from build123d import *

# Parameters (mm, degrees)
F1_DEPTH = 482.6
F2_R     = 22.9562722026
F3_DEPTH = 25.4


# Not quite as in the source:
# - a feature names something its author has since deleted; it is built from what else it names


with BuildPart() as f1:
    # F0 (on Right) → F1 (new body)
    with BuildSketch(Plane.YZ):
        with BuildLine():
            Line((-812.6182556152, 512.6869344869), (-812.6182556152, 611.3093582153))
            Line((-812.6182556152, 611.3093582153), (-825.3182556152, 611.3093582153))
            Line((-825.3182556152, 611.3093582153), (-825.3182556152, 510.914683342))
            ThreePointArc((-825.3182556152, 510.914683342), (-828.5785642638, 501.8659167533), (-836.8610188459, 496.9760562897))
            Line((-836.8610188459, 496.9760562897), (-938.4610188459, 496.9760562897))
            Line((-938.4610188459, 496.9760562897), (-938.4610188459, 484.2760562897))
            Line((-938.4610188459, 484.2760562897), (-840.6965225196, 484.2760562897))
            ThreePointArc((-840.6965225196, 484.2760562897), (-822.0453350188, 489.7370832304), (-812.6182556152, 506.7317819438))
            ThreePointArc((-812.6182556152, 506.7317819438), (-812.7921868823, 509.7093582153), (-812.6182556152, 512.6869344869))
        make_face()
    extrude(amount=F1_DEPTH)

    # F2 (on Right) → F3 (join)
    with BuildSketch(Plane.YZ):
        with Locations((-826.0604739189, 499.5044767857)):
            Circle(F2_R)
    extrude(amount=F3_DEPTH)


solid = f1.part
The model under review builds one solid part; all positions refer to its coordinate system, in mm. A direction names the side the tool comes from. Coordinates: 2 decimals unless noted, no trailing zeros. Order: outer loops, then holes, each group sorted by start corner. A loop starts at its lowest first (then second) coordinate and runs counter-clockwise, first axis right, second up. Notation, with made-up numbers: (-11, 1) -> (44, 1) arc R29 cw to (44, 30) -> close; hole circle Ø3 at (8.25, -36.5). An arc over 180 degrees is marked (long way). Answer in a Markdown table with one row per item.
(1) Machinability: for faces 1 (the flat face through (238, -938.461, 491)), 2 (the flat face through (25.4, -837, 510)), which of the approach directions +Z, -Z, +X, -X, +Y, -Y give a long, thin tool a straight path to every point of the face, cutting with its end or side? Answer none if there is none.
Answers:
| item | result |
|---|---|
| face 1 | +Z, -Z, +X, -X, -Y |
| face 2 | +Z, +X, -Y |
(2) Insertion check: pin 1 (3 mm diameter, centred on x = 188, z = 578, fed in from -Y); pin 2 (3 mm diameter, centred on x = 112, y = -870, fed in from -Z); pin 3 (8 mm diameter, centred on x = 218, z = 507, fed in from +Y). Each pin has a flat end and moves straight along its axis. Give the tip position at first contact, or say it passes through.
Answers:
| item | result |
|---|---|
| pin 1 | y = -825.32 |
| pin 2 | z = 484.28 |
| pin 3 | y = -812.62 |
(3) Consider section A-A (x = 370.5). Write out the cut boundary in (y, z).
Answers:
| item | result |
|---|---|
| outline | (-938.46, 484.28) -> (-840.7, 484.28) arc R25.57 ccw to (-812.62, 506.73) arc R25.57 cw to (-812.62, 512.69) -> (-812.62, 611.31) -> (-825.32, 611.31) -> (-825.32, 510.91) arc R14.19 cw to (-836.86, 496.98) -> (-938.46, 496.98) -> close |
(4) Consider section B-B (z = 592). Write out the cut boundary in (x, y), plus the area to 3 significant figures.
Answers:
| item | result |
|---|---|
| outline | (0, -825.32) -> (482.6, -825.32) -> (482.6, -812.62) -> (0, -812.62) -> close |
| area | 6,130 mm² |
(5) Wall thickness on line 1 along Y through (x, z) = (344.5, 589); line 2 along Z through (x, y) = (197, -886); line 3 along Y through (x, z) = (440, 509.5): over which ranges is each line inside the solid? List them lowest first.
Answers:
| item | result |
|---|---|
| line 1 | -825.32 to -812.62 |
| line 2 | 484.28 to 496.98 |
| line 3 | -825.39 to -812.79 |
(6) Consider section C-C (y = -899.5). Write out the cut boundary in (x, z).
Answers:
| item | result |
|---|---|
| outline | (0, 484.28) -> (482.6, 484.28) -> (482.6, 496.98) -> (0, 496.98) -> close |
